Work out the finished part from the listing and answer in its coordinate system (mm). Face numbers are marked on the shaded views. A direction names the side the tool comes from. Give positions to 0.01 mm unless a question says otherwise; leave off trailing zeros. Order: outer loops, then holes, each group sorted by start corner. A loop starts at its lowest first (then second) coordinate and runs counter-clockwise, first axis right, second up. Notation, with made-up numbers: (11, -18.75) -> (48, -18.75) arc R20 ccw to (48, -12.75) -> close; hole circle Ø10 at (47.5, 24.25). An arc over 180 degrees is marked (long way). Answer as CSV lines item,"result". Start each with the question number.
1. For a pull along X with two mould halves and no side action, classify the marked faces 1, 2, 3 and 4 as released by +X, released by -X, zero draft, split by the parting line, or undercut.
2. A cutting plane is placed at C-C (y = 2.5). Give the vertices of the cut face in (x, z) (3 decimals).
3. For the marked faces 5 and 6, determine the directions among +Z, -Z, +X, -X, +Y, -Y from which every point of the face is accessible in a straight line to the end or side of a thin tool.
4. A cutting plane is placed at B-B (x = 25.4). Give the vertices of the cut face in (y, z).
5. A cutting plane is placed at D-D (z = 0.5). Give the vertices of the cut face in (x, y) (3 decimals).
6. Flat-ended cylindrical pins translate along their axes: pin 1 (1.9 mm diameter, centred on x = 25.4, y = 3.175, fed in from -Z); pin 2 (1.9 mm diameter, centred on x = 13, y = 4.5, fed in from +Z) (3 decimals); pin 3 (1.6 mm diameter, centred on y = 1.5, z = 5.5, fed in from -X). Find the tip coordinate at first contact, or state that the pin passes through.
7. Find the intervals of material crossed by L1, parallel to X at y = 2.25, z = 1 (3 decimals); L2, parallel to Y at x = 25.4, z = 2.5; L3, parallel to X at y = 2.5, z = 1.5 (3 decimals), in increasing order.
8. A cutting plane is placed at A-A (z = 4). Give the vertices of the cut face in (x, y) (3 decimals), then the cut area to 3 significant figures.
from build123d import *

# Parameters (mm, degrees)
F0_W     = 6.35
F0_H     = 6.35
F0_R     = 1.1751262937
F1_DEPTH = 6.35
F0_W_2   = 7.9375
F2_DEPTH = 3.175


with BuildPart() as f1:
    # F0 (on Top) → F1 (new body)
    with BuildSketch(Plane.XY):
        with Locations((3.175, 3.175)):
            Rectangle(F0_W, F0_H)
        with Locations((3.175, 3.175)):
            Circle(F0_R, mode=Mode.SUBTRACT)
    extrude(amount=F1_DEPTH)



with BuildPart() as f1b:
    # F0 (on Top) → F1, piece 2 (new body)
    with BuildSketch(Plane.XY):
        with Locations((25.4, 3.175)):
            Rectangle(F0_W, F0_H)
        with Locations((25.4, 3.175)):
            Circle(F0_R, mode=Mode.SUBTRACT)
    extrude(amount=F1_DEPTH)


with BuildPart() as f1_1:
    add(f1.part)

    add(f1b.part)  # F2 merges F1b
    # F0 (on Top) → F2 (join)
    with BuildSketch(Plane.XY):
        with Locations((10.31875, 3.175)):
            Rectangle(F0_W_2, F0_H)
        with Locations((18.25625, 3.175)):
            Rectangle(F0_W_2, F0_H)
    extrude(amount=F2_DEPTH)


solid = f1_1.part
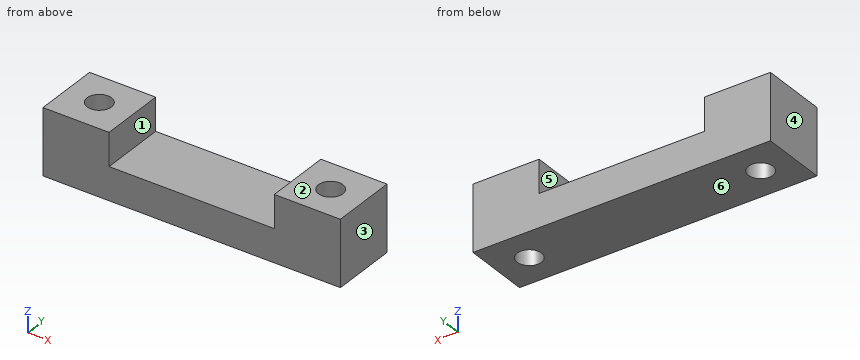
Answer sheet:
1,face 1,"undercut"
1,face 2,"zero draft"
1,face 3,"released by +X"
1,face 4,"released by -X"
2,outline,"(0, 0) -> (2.213, 0) -> (2.213, 6.35) -> (0, 6.35) -> close; (4.137, 0) -> (24.438, 0) -> (24.438, 6.35) -> (22.225, 6.35) -> (22.225, 3.175) -> (6.35, 3.175) -> (6.35, 6.35) -> (4.137, 6.35) -> close; (26.362, 0) -> (28.575, 0) -> (28.575, 6.35) -> (26.362, 6.35) -> close"
3,face 5,"+Z, +Y, -Y"
3,face 6,"-Z, +X, -X, +Y, -Y"
4,outline,"(0, 0) -> (2, 0) -> (2, 6.35) -> (0, 6.35) -> close; (4.35, 0) -> (6.35, 0) -> (6.35, 6.35) -> (4.35, 6.35) -> close"
5,outline,"(0, 0) -> (28.575, 0) -> (28.575, 6.35) -> (0, 6.35) -> close; hole circle Ø2.35 at (3.175, 3.175); hole circle Ø2.35 at (25.4, 3.175)"
6,pin 1,"passes through"
6,pin 2,"stops at z = 3.175"
6,pin 3,"stops at x = 0"
7,L1,"x = 0 to 2.45, 3.9 to 24.675, 26.125 to 28.575"
7,L2,"y = 0 to 2, 4.35 to 6.35"
7,L3,"x = 0 to 2.213, 4.137 to 24.438, 26.362 to 28.575"
8,outline,"(0, 0) -> (6.35, 0) -> (6.35, 6.35) -> (0, 6.35) -> close; (22.225, 0) -> (28.575, 0) -> (28.575, 6.35) -> (22.225, 6.35) -> close; hole circle Ø2.35 at (3.175, 3.175); hole circle Ø2.35 at (25.4, 3.175)"
8,area,"72.0 mm^2"
